from build123d import *

# Parameters (mm, degrees)
F2_R = 0.59


with BuildPart() as f1:
    # F0 (on Right) → F1 (revolve)
    with BuildSketch(Plane.YZ):
        Polygon((0, 5), (0, 1.5), (3.5, 1.5), (3.5, 5), (2.5, 5), (2.25, 3.5), (1.25, 3.5), (1, 5), align=None)
    revolve(axis=Axis((0, 1.75, 0), (0, 1, 0)))

    # F2
    f2_edges = [f1.edges().sort_by_distance(p)[0] for p in [
        (0, 1.25, -3.5),
        (0, 1, -5),
        (0, 1.125, 4.25),
        (0, 2.5, -5),
        (0, 2.25, -3.5),
        (0, 2.375, 4.25),
    ]]
    fillet(f2_edges, radius=F2_R)


solid = f1.part
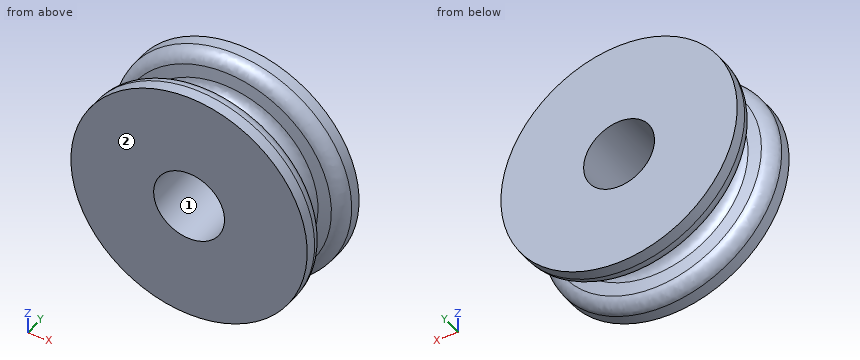
Read the model definition and answer for the solid it produces. Units are mm, in the model's axes. Face numbers are marked on the shaded views. Round coordinates to 2 decimals unless told otherwise and drop trailing zeros. Order: outer loops, then holes, each group sorted by start corner. A loop starts at its lowest first (then second) coordinate and runs counter-clockwise, first axis right, second up.
1) The part is cut by section A-A on y = 3.2. Write down the section's boundary in (x, z).
2) Straight lines are drawn through the part: L1, parallel to Y at x = 4.5, z = 2; L2, parallel to Y at x = 4.5, z = 1; L3, parallel to Z at x = -1, y = 1.65. For each, find the intervals that lie inside material, in ascending order.
3) Flat-ended cylindrical pins translate along their axes: pin 1 (3 mm diameter, centred on x = 4, z = -1, fed in from -Y); pin 2 (2 mm diameter, centred on y = 3, z = 3.5, fed in from -X). Find the tip coordinate at first contact, or state that the pin passes through.
4) The mould has two halves that part along X. Classify the marked faces 1 and 2: released by +X, released by -X, zero draft, split by the parting line, or undercut.
Resolved:
1. outline: circle Ø10 at (0, 0); hole circle Ø3 at (0, 0)
2. L1: y = 0 to 0.79, 2.71 to 3.5
2. L2: y = 0 to 1.06, 2.44 to 3.5
2. L3: z = -3.36 to -1.12, 1.12 to 3.36
3. pin 1: stops at y = 0
3. pin 2: stops at x = -4.33
4. face 1: undercut
4. face 2: zero draft
